```python
from build123d import *

# Parameters (mm, degrees)
SKETCH1_R                 = 114.3
SKETCH1_R_2               = 76.2
BOSS_EXTRUDE1_DEPTH       = 5.969
SKETCH2_R                 = 3.175
CUT_EXTRUDE1_DEPTH        = 12.7
CIRPATTERN5_COUNT         = 20
SKETCH9_R                 = 4.5
BOSS_EXTRUDE4_DEPTH       = 5.969
FILLET1_R                 = 6.35
CIRPATTERN8_COUNT         = 5
FILLET1_OF_CIRPATTERN8_R  = 6.35
SKETCH14_R                = 76.2
SKETCH14_R_2              = 34.925
BOSS_EXTRUDE6_DEPTH       = 5.969
SKETCH16_R                = 4.5
CUT_EXTRUDE3_DEPTH        = 5.969
CIRPATTERN9_COUNT         = 5
SKETCH17_R                = 66.675
SKETCH17_R_2              = 6.88
CUT_EXTRUDE4_DEPTH        = 5.969
CIRPATTERN10_COUNT        = 4
CUT_EXTRUDE6_DEPTH        = 162.754780334
FILLET2_R                 = 10
CIRPATTERN11_COUNT        = 4
FILLET2_OF_CIRPATTERN11_R = 10


with BuildPart() as part:
    # Sketch1 → Boss-Extrude1 (new body)
    with BuildSketch(Plane.XY):
        Circle(SKETCH1_R)
        Circle(SKETCH1_R_2, mode=Mode.SUBTRACT)
    extrude(amount=BOSS_EXTRUDE1_DEPTH)

    # Sketch2 → Cut-Extrude1 (cut)
    with BuildSketch(Plane.XY.offset(5.969)):
        with Locations((-37.394976935, 97.79)):
            Circle(SKETCH2_R)
        with Locations((-27.49630657, 92.075)):
            Circle(SKETCH2_R)
        with Locations((-17.597636205, 86.36)):
            Circle(SKETCH2_R)
    cut_extrude1 = extrude(amount=-CUT_EXTRUDE1_DEPTH, mode=Mode.SUBTRACT)

    # CirPattern5: Cut-Extrude1 ×20 about axis
    cirpattern5_axis = Axis((0, 0, 0), (0, 0, 1))
    for i in range(1, CIRPATTERN5_COUNT):
        add(cut_extrude1.rotate(cirpattern5_axis, i * 360 / CIRPATTERN5_COUNT), mode=Mode.SUBTRACT)

    # Sketch9 → Boss-Extrude4 (add)
    with BuildSketch(Plane(origin=(0, 0, 0), x_dir=(-1, 0, 0), z_dir=(0, 0, -1))):
        with BuildLine():
            Line((7.427010516, 41.456201743), (12.172412147, 75.221488835))
            ThreePointArc((12.172412147, 75.221488835), (0, 76.2), (-12.172412147, 75.221488835))
            Line((-12.172412147, 75.221488835), (-7.427010516, 41.456201743))
            ThreePointArc((-7.427010516, 41.456201743), (0, 35), (7.427010516, 41.456201743))
        make_face()
        with Locations((0, 42.5)):
            Circle(SKETCH9_R, mode=Mode.SUBTRACT)
    boss_extrude4 = extrude(amount=-BOSS_EXTRUDE4_DEPTH)

    # Fillet1
    fillet1_edges = [part.edges().sort_by_distance(p)[0] for p in [
        (12.172412147, 75.221488835, 2.9845),
        (-12.172412147, 75.221488835, 2.9845),
    ]]
    fillet(fillet1_edges, radius=FILLET1_R)

    # CirPattern8: Boss-Extrude4 ×5 about axis
    cirpattern8_axis = Axis((0, 0, 0), (0, 0, 1))
    for i in range(1, CIRPATTERN8_COUNT):
        add(boss_extrude4.rotate(cirpattern8_axis, i * 360 / CIRPATTERN8_COUNT))

    # Fillet1 of CirPattern8
    fillet1_of_cirpattern8_edges = [part.edges().sort_by_distance(p)[0] for p in [
        (-67.778404906, 34.821370284, 2.9845),
        (-75.301369338, 11.6680665, 2.9845),
        (-54.061770082, -53.700698464, 2.9845),
        (-34.366393503, -68.010227155, 2.9845),
        (34.366393503, -68.010227155, 2.9845),
        (54.061770082, -53.700698464, 2.9845),
        (75.301369338, 11.6680665, 2.9845),
        (67.778404906, 34.821370284, 2.9845),
    ]]
    fillet(fillet1_of_cirpattern8_edges, radius=FILLET1_OF_CIRPATTERN8_R)

    # Sketch14 → Boss-Extrude6 (add)
    with BuildSketch(Plane.XY):
        Circle(SKETCH14_R)
        Circle(SKETCH14_R_2, mode=Mode.SUBTRACT)
    extrude(amount=BOSS_EXTRUDE6_DEPTH)

    # Sketch16 → Cut-Extrude3 (cut)
    with BuildSketch(Plane.XY):
        with Locations((0, 42.5)):
            Circle(SKETCH16_R)
    cut_extrude3 = extrude(amount=CUT_EXTRUDE3_DEPTH, mode=Mode.SUBTRACT)

    # CirPattern9: Cut-Extrude3 ×5 about axis
    cirpattern9_axis = Axis((0, 0, 0), (0, 0, 1))
    for i in range(1, CIRPATTERN9_COUNT):
        add(cut_extrude3.rotate(cirpattern9_axis, i * 360 / CIRPATTERN9_COUNT), mode=Mode.SUBTRACT)

    # Sketch17 → Cut-Extrude4 (cut)
    with BuildSketch(Plane(origin=(0, 0, 0), x_dir=(-1, 0, 0), z_dir=(0, 0, -1))):
        Circle(SKETCH17_R)
        with Locations((-33.3375, 57.742243797)):
            Circle(SKETCH17_R_2)
        with Locations((-57.742243797, 33.3375)):
            Circle(SKETCH17_R_2)
    cut_extrude4 = extrude(amount=-CUT_EXTRUDE4_DEPTH, mode=Mode.SUBTRACT)

    # CirPattern10: Cut-Extrude4 ×4 about axis
    cirpattern10_axis = Axis((0, 0, 0), (0, 0, 1))
    for i in range(1, CIRPATTERN10_COUNT):
        add(cut_extrude4.rotate(cirpattern10_axis, i * 360 / CIRPATTERN10_COUNT), mode=Mode.SUBTRACT)

    # Sketch19 → Cut-Extrude6 (cut, through all)
    with BuildSketch(Plane(origin=(0, 0, 0), x_dir=(-1, 0, 0), z_dir=(0, 0, -1))):
        with BuildLine():
            Line((-19.722011237, 73.603547963), (-17.256759832, 64.403104468))
            ThreePointArc((-17.256759832, 64.403104468), (-8.702833866, 66.104586132), (0, 66.675))
            Line((0, 66.675), (0, 76.2))
            ThreePointArc((0, 76.2), (-9.946095847, 75.548098437), (-19.722011237, 73.603547963))
        make_face()
        with BuildLine():
            ThreePointArc((0, 66.675), (8.702833866, 66.104586132), (17.256759832, 64.403104468))
            Line((17.256759832, 64.403104468), (19.722011237, 73.603547963))
            ThreePointArc((19.722011237, 73.603547963), (9.946095847, 75.548098437), (0, 76.2))
            Line((0, 76.2), (0, 66.675))
        make_face()
    cut_extrude6 = extrude(amount=-CUT_EXTRUDE6_DEPTH, mode=Mode.SUBTRACT)

    # Fillet2
    # the kernel refuses this fillet: 10 mm, written as the material it adds along each edge
    with BuildSketch(Plane(origin=(-19.722011237, 73.603547963, 0), x_dir=(0.982649179352288, 0.18547396129450383, 0), z_dir=(0, 0, 1))) as fillet2_piece_1:
        with BuildLine():
            CenterArc((10.704810772, -9.971704141), FILLET2_R, 85.688766621, 91.596368931)
            Line((0.716034569, -9.498048194), (0.516259045, -9.488575075))
            ThreePointArc((0.516259045, -9.488575075), (0.158583202, -4.764058944), (-0.199434083, -0.015034847))
            Line((-0.199434083, -0.015034847), (-0.015034847, 0.199434083))
            ThreePointArc((-0.015034847, 0.199434083), (5.728276551, 0.415614448), (11.471587949, 0.199434083))
            Line((11.471587949, 0.199434083), (11.456553102, 0))
        make_face()
    extrude(amount=5.969)
    with BuildSketch(Plane(origin=(19.722011237, 73.603547963, 0), x_dir=(-0.2588190451025574, -0.9659258262890585, 0), z_dir=(0, 0, 1))) as fillet2_piece_2:
        with BuildLine():
            CenterArc((10.748214286, -9.92490538), FILLET2_R, 97.026097827, 91.596368931)
            Line((0.861237592, -11.4241358), (0.663498058, -11.454120409))
            ThreePointArc((0.663498058, -11.454120409), (0.016180365, -5.743311398), (-0.2, 0))
            Line((-0.2, 0), (0, 0.2))
            ThreePointArc((0, 0.2), (4.7625, 0.2), (9.500535714, 0.198498108))
            Line((9.500535714, 0.198498108), (9.525, 0))
        make_face()
    extrude(amount=5.969)

    # CirPattern11: Cut-Extrude6 ×4 about axis
    cirpattern11_axis = Axis((0, 0, 0), (0, 0, 1))
    for i in range(1, CIRPATTERN11_COUNT):
        add(cut_extrude6.rotate(cirpattern11_axis, i * 360 / CIRPATTERN11_COUNT), mode=Mode.SUBTRACT)

    # Fillet2 of CirPattern11
    # the kernel refuses this fillet: 10 mm, written as the material it adds along each edge
    with BuildSketch(Plane(origin=(-73.603547963, -19.722011237, 0), x_dir=(0.9659258262890572, 0.2588190451025623, 0), z_dir=(0, 0, 1)), Plane(origin=(19.722011237, -73.603547963, 0), x_dir=(-0.2588190451025616, 0.9659258262890574, 0), z_dir=(0, 0, 1)), Plane(origin=(73.603547963, 19.722011237, 0), x_dir=(-0.9659258262890574, -0.2588190451025616, 0), z_dir=(0, 0, 1))) as fillet2_of_cirpattern11_piece_1:
        with BuildLine():
            CenterArc((10.748214286, 9.92490538), FILLET2_OF_CIRPATTERN11_R, 171.377533242, 91.596368931)
            Line((0.861237592, 11.4241358), (0.663498058, 11.454120409))
            ThreePointArc((0.663498058, 11.454120409), (0.016180365, 5.743311398), (-0.2, 0))
            Line((-0.2, 0), (0, -0.2))
            ThreePointArc((0, -0.2), (4.7625, -0.2), (9.500535714, -0.198498108))
            Line((9.500535714, -0.198498108), (9.525, 0))
        make_face()
    extrude(amount=5.969)
    with BuildSketch(Plane(origin=(-73.603547963, 19.722011237, 0), x_dir=(-0.18547396129450153, -0.9826491793522883, 0), z_dir=(0, 0, 1)), Plane(origin=(-19.722011237, -73.603547963, 0), x_dir=(0.9826491793522883, -0.18547396129450153, 0), z_dir=(0, 0, 1)), Plane(origin=(73.603547963, -19.722011237, 0), x_dir=(0.18547396129450147, 0.9826491793522883, 0), z_dir=(0, 0, 1))) as fillet2_of_cirpattern11_piece_2:
        with BuildLine():
            CenterArc((10.704810772, 9.971704141), FILLET2_OF_CIRPATTERN11_R, 182.714864448, 91.596368931)
            Line((0.716034569, 9.498048194), (0.516259045, 9.488575075))
            ThreePointArc((0.516259045, 9.488575075), (0.158583202, 4.764058944), (-0.199434083, 0.015034847))
            Line((-0.199434083, 0.015034847), (-0.015034847, -0.199434083))
            ThreePointArc((-0.015034847, -0.199434083), (5.728276551, -0.415614448), (11.471587949, -0.199434083))
            Line((11.471587949, -0.199434083), (11.456553102, 0))
        make_face()
    extrude(amount=5.969)


solid = part.part
```
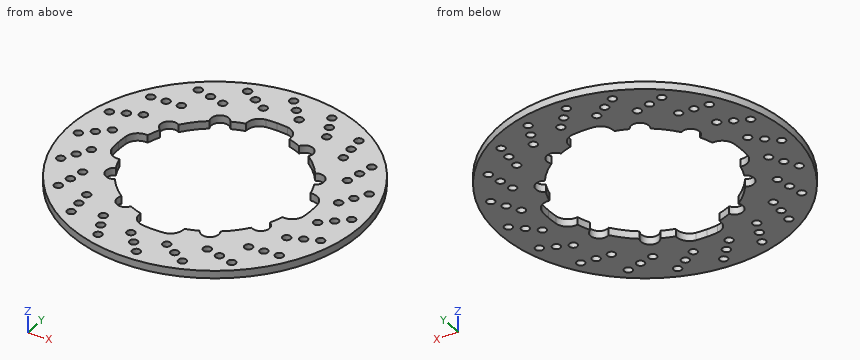
CAD build for the part. Positions are in the model's coordinates, mm. Round coordinates to 2 decimals unless told otherwise and drop trailing zeros.
Item 1: Saw through at A-A on z = 3.8. State how many separate pieces and enclosed holes the cut face has, then the cut area to 3 significant figures.
Item 2: Probe line 1 along X through (y, z) = (-2, 5.65); line 2 along X through (y, z) = (19.5, 3.35); line 3 along X through (y, z) = (75, 4.4). List the from-to ranges inside material, lowest first.
Item 3: Pin check, flat tips, straight feed: pin 1 (5.5 mm diameter, centred on x = -31.88, y = -90.65, fed in from +Z); pin 2 (2 mm diameter, centred on x = 18.5, z = 4, fed in from -Y); pin 3 (1 mm diameter, centred on y = 34, z = 3.5, fed in from -X); pin 4 (1.5 mm diameter, centred on y = -86.5, z = 1.5, fed in from +X). Stop position of each tip, or through.
Reported:
1. separate pieces: 1
1. enclosed holes: 61
1. area: 23,400 mm2
2. line 1: x = -114.28 to -76.17, 76.17 to 92.9, 99.23 to 114.28
2. line 2: x = -112.62 to -63.76, 63.76 to 83.82, 88.9 to 112.62
2. line 3: x = -86.25 to -46.11, -40.74 to -11.25, 11.25 to 55.46, 61.19 to 86.25
3. pin 1: passes through
3. pin 2: stops at y = -112.95
3. pin 3: stops at x = -109.28
3. pin 4: stops at x = 75.57
